Here's how the part is built. I have some questions about the finished solid (model axes, mm). Face numbers are marked on the shaded views. Give positions to 0.01 mm unless a question says otherwise; leave off trailing zeros. Write each loop counter-clockwise with the first axis right and the second up, starting at its lowest first coordinate (ties: lowest second). Pieces come first, ordered by that corner, then holes. Notation, with made-up numbers: (48, 63.5) - (60, 63.5) arc R30 cw to (60, 97.5) - close; hole circle Ø8 at (6, -1). An arc over 180 degrees is marked (long way). Use one line per item in the form item = value. Start each with the question number.
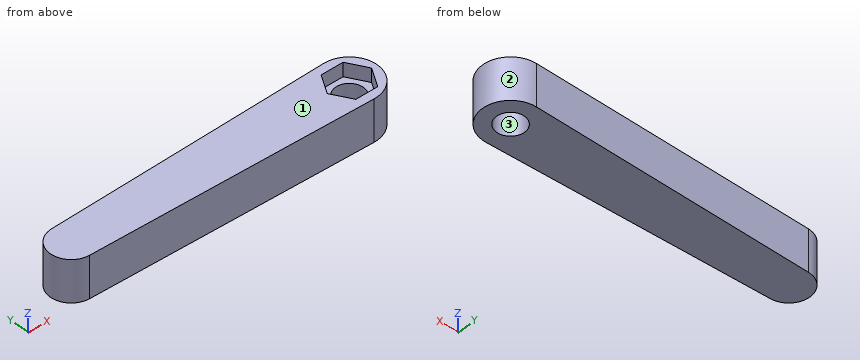
Autodesk Inventor part; units mm, degrees
ref_plane "YZ Plane" through (0, 0, 0) normal (1, 0, 0) x (0, 1, 0)
ref_plane "XZ Plane" through (0, 0, 0) normal (0, 1, 0) x (-1, 0, 0)
ref_plane "XY Plane" through (0, 0, 0) normal (0, 0, 1) x (1, 0, 0)
sketch "Boceto1" plane through (0, 0, 0) normal (0, 0, 1) x (1, 0, 0)
  arc A0 (-0.1, -3.9987) -> (-0.1, 3.9987) centre (0, 0) ccw
  line L0 (0, 0) -> (-40, 0)
  arc A1 (-40.075, 2.9991) -> (-40.075, -2.9991) centre (-40, 0) ccw
  line L1 (-40.075, 2.9991) -> (-0.1, 3.9987)
  line L2 (-40.075, -2.9991) -> (-0.1, -3.9987)
  dimension "d0" = 8
  dimension "d1" = 40
  dimension "d2" = 6
extrude "Extrusión1" add sketch "Boceto1" along normal blind 6
sketch "Boceto2" plane through (0, 0, 6) normal (0, 0, 1) x (1, 0, 0)
  arc A0 (-0.1, -3.9987) -> (-0.1, 3.9987) centre (0, 0) ccw
hole "Agujero1" at (0, 0, 6) direction (0, 0, -1) diameter 4 depth 11.75 tip angle 118
sketch "Boceto3" plane through (0, 0, 6) normal (0, 0, 1) x (1, 0, 0)
  line L0 (-1.5877, 2.75) -> (1.5877, 2.75)
  line L1 (1.5877, 2.75) -> (3.1754, 0)
  line L2 (3.1754, 0) -> (1.5877, -2.75)
  line L3 (1.5877, -2.75) -> (-1.5877, -2.75)
  line L4 (-1.5877, -2.75) -> (-3.1754, 0)
  line L5 (-3.1754, 0) -> (-1.5877, 2.75)
  point P0 (0, 0)
  point P1 (0, 0)
  dimension "d12" = 5.5
extrude "Extrusión2" cut sketch "Boceto3" against normal blind 2
properties part number "Brazo"
1. I want a section at C-C, the plane z = 4.95. List the corners of the cut face in (x, y) for me (3 decimals), then the cut area to 3 significant figures.
2. Please list where these lines run through material, in increasing order: line 1 (Y direction, x = 0, z = 2.5); line 2 (X direction, y = -0.75, z = 4.45); line 3 (Y direction, x = -0.5, z = 2.45).
3. For P1, Ø3, axis at x = 0, y = 0, coming from the +Z side; P2, Ø1, axis at x = -9.5, z = 5.5, coming from the +Y side; P3, Ø0.6, axis at x = -0.5, z = 5, coming from the +Y side; P4, Ø1, axis at y = 3, z = 1.5, coming from the +X side, each with a flat end and sliding along its axis, tell me the tip position at first contact or that it passes through.
4. We'd pull the mould along Y, two halves only. Please class the marked faces 1, 2 and 3: pulls with the +Y half, pulls with the -Y half, needs draft (parallel to the pull), parting line crosses it, or undercut.
5. I want a section at B-B, the plane y = -0.75. List the corners of the cut face in (x, z) for me, then the cut area to 3 significant figures.
6. I want a section at A-A, the plane z = 2.6. List the corners of the cut face in (x, y) for me (3 decimals), then the cut area to 3 significant figures.
7. I want a section at D-D, the plane x = -10.5. List the corners of the cut face in (y, z) for me, then the cut area to 3 significant figures.
Result sheet:
q1.outline = (-40.075, -2.999) - (-0.1, -3.999) arc R4 ccw (long way) to (-0.1, 3.999) - (-40.075, 2.999) arc R3 ccw to start; hole (-3.175, 0) - (-1.588, -2.75) - (1.588, -2.75) - (3.175, 0) - (1.588, 2.75) - (-1.588, 2.75) - close
q1.area = 293 mm2
q2.line_1 = -4 to -2, 2 to 4
q2.line_2 = -42.9 to -2.74, 2.74 to 3.93
q2.line_3 = -3.99 to -1.94, 1.94 to 3.99
q3.P1 = through
q3.P2 = 3.78
q3.P3 = 4
q3.P4 = 3.12
q4.face_1 = needs draft
q4.face_2 = parting line crosses it
q4.face_3 = undercut
q5.outline = (-42.9, 0) - (-1.85, 0) - (-1.85, 4) - (-2.74, 4) - (-2.74, 6) - (-42.9, 6) - close; (1.85, 0) - (3.93, 0) - (3.93, 6) - (2.74, 6) - (2.74, 4) - (1.85, 4) - close
q5.area = 255 mm2
q6.outline = (-40.075, -2.999) - (-0.1, -3.999) arc R4 ccw (long way) to (-0.1, 3.999) - (-40.075, 2.999) arc R3 ccw to start; hole circle Ø4 at (0, 0)
q6.area = 307 mm2
q7.outline = (-3.74, 0) - (3.74, 0) - (3.74, 6) - (-3.74, 6) - close
q7.area = 44.9 mm2
